Verification items for the finished model (mm, model axes). A direction names the side the tool comes from. Round coordinates to 2 decimals unless told otherwise and drop trailing zeros. Write each loop counter-clockwise with the first axis right and the second up, starting at its lowest first coordinate (ties: lowest second). Pieces come first, ordered by that corner, then holes. Notation, with made-up numbers: (45, -35.75) - (90, -35.75) arc R27 cw to (90, -3.75) - close; hole circle Ø9 at (26, 52.5). An arc over 180 degrees is marked (long way). Answer as a JSON object with one key per item and string values. Group by question number.
1) Set-up check for faces 4 (the flat face through (8.5, 10, 17)), 5 (the flat face through (2, 35, -11.5)): record each of +Z, -Z, +X, -X, +Y, -Y from which the full face is reachable in a straight line by a thin tool's end or side.
2) Section check C-C (x = 1.25). Enter the section's corners in (y, z).
3) Section check A-A (z = 18). Enter the section's corners in (x, y), then the cut area to 3 significant figures.
4) Thickness scan on line 1 (Y direction, x = 1.75, z = 0); line 2 (Y direction, x = -2.5, z = 0.5); line 3 (Z direction, x = -6.5, y = -2.5). Record the ranges inside material, lowest first.
5) Section check B-B (y = 42). Enter the section's corners in (x, z), then the cut area to 3 significant figures.
6) Mould release check, pull along Z, two halves, no side actions. Record for faces 1 (the cylindrical face through (0.119, -19.961, -10.382)), 2 (the flat face through (2, 35, 11.5)), 3 (the cylindrical face through (1.99, 34.11, -1.34)): +Z half, -Z half, draft (parallel to the pull), parting line (faces both ways), or undercut.
7) Section check D-D (z = 0). Enter the section's corners in (x, y), then the cut area to 3 significant figures.
8) Go/stop test with flat-tipped pins: pin 1 Ø2 at (x, z) = (5, 16) entering from +Y; pin 2 Ø3 at (x, z) = (-3.5, -6) entering from -Y; pin 3 Ø1.5 at (y, z) = (36.5, 5) entering from +X. Record where each tip stops, or that it passes through.
```python
from build123d import *

# Parameters (mm, degrees)
SKETCH2_R                = 22.5
BOSS_EXTRUDE1_DEPTH      = 8.5
BOSS_EXTRUDE2_REACH      = 78.386
BOSS_EXTRUDE2_END_RADIUS = 22.5
SKETCH3_W                = 10
SKETCH3_H                = 23
SKETCH8_R                = 2.5
CUT_EXTRUDE1_DEPTH       = 57.95722287
SKETCH11_R               = 19.5
CUT_EXTRUDE2_DEPTH       = 58.404268134


with BuildPart() as part:
    # Sketch2 → Boss-Extrude1 (new, symmetric)
    with BuildSketch(Plane(origin=(0, 0, 0), x_dir=(0, 0, -1), z_dir=(1, 0, 0))):
        Circle(SKETCH2_R)
    extrude(amount=BOSS_EXTRUDE1_DEPTH, both=True)

    # Boss-Extrude2: up to this cylinder (the profile starts outside it)
    boss_extrude2_end = Plane(origin=(1.923205, 0, 0), z_dir=(-1, 0, 0)) * Cylinder(BOSS_EXTRUDE2_END_RADIUS, 202.772, mode=Mode.PRIVATE)
    # Sketch3 → Boss-Extrude2 (add, up to the surface)
    with BuildSketch(Plane(origin=(0, 50, 0), x_dir=(1, 0, 0), z_dir=(0, 1, 0)), mode=Mode.PRIVATE) as boss_extrude2_sk1:
        with Locations((1.9232045, 0)):
            Rectangle(SKETCH3_W, SKETCH3_H)
    boss_extrude2_tool1 = extrude(boss_extrude2_sk1.sketch, amount=-BOSS_EXTRUDE2_REACH, mode=Mode.PRIVATE) - boss_extrude2_end
    add(boss_extrude2_tool1.solids().sort_by_distance((1.923205, 50, 0))[0])

    # Sketch8 → Cut-Extrude1 (cut, through all)
    with BuildSketch(Plane(origin=(6.9232045, 0, 0), x_dir=(0, 0, -1), z_dir=(1, 0, 0))):
        with Locations((0, 42)):
            Circle(SKETCH8_R)
        with Locations((0, 32)):
            Circle(SKETCH8_R)
    extrude(amount=-CUT_EXTRUDE1_DEPTH, mode=Mode.SUBTRACT)

    # Sketch11 → Cut-Extrude2 (cut, through all)
    with BuildSketch(Plane(origin=(8.5, 0, 0), x_dir=(0, 0, -1), z_dir=(1, 0, 0))):
        Circle(SKETCH11_R)
    extrude(amount=-CUT_EXTRUDE2_DEPTH, mode=Mode.SUBTRACT)


solid = part.part
```
Returned:
{
 "1": {"face 4": "+Z, -Z, +X, +Y, -Y", "face 5": "-Z, +X, -X, +Y"},
 "2": {"outline": "(19.34, -11.5) - (50, -11.5) - (50, 11.5) - (19.34, 11.5) arc R22.5 ccw (long way) to start; hole circle Ø39 at (0, 0); hole circle Ø5 at (32, 0); hole circle Ø5 at (42, 0)"},
 "3": {"outline": "(-8.5, -13.5) - (8.5, -13.5) - (8.5, -7.5) - (-8.5, -7.5) - close; (-8.5, 7.5) - (8.5, 7.5) - (8.5, 13.5) - (-8.5, 13.5) - close", "area": "204 mm2"},
 "4": {"line 1": "-22.5 to -19.5, 19.5 to 29.5, 34.5 to 39.5, 44.5 to 50", "line 2": "-22.49 to -19.49, 19.49 to 29.55, 34.45 to 39.55, 44.45 to 50", "line 3": "-22.36 to -19.34, 19.34 to 22.36"},
 "5": {"outline": "(-3.08, -11.5) - (6.92, -11.5) - (6.92, -2.5) - (-3.08, -2.5) - close; (-3.08, 2.5) - (6.92, 2.5) - (6.92, 11.5) - (-3.08, 11.5) - close", "area": "180 mm2"},
 "6": {"face 1": "parting line", "face 2": "+Z half", "face 3": "undercut"},
 "7": {"outline": "(-8.5, -22.5) - (8.5, -22.5) - (8.5, -19.5) - (-8.5, -19.5) - close; (-8.5, 19.5) - (8.5, 19.5) - (8.5, 22.5) - (6.92, 22.5) - (6.92, 29.5) - (-3.08, 29.5) - (-3.08, 22.5) - (-8.5, 22.5) - close; (-3.08, 34.5) - (6.92, 34.5) - (6.92, 39.5) - (-3.08, 39.5) - close; (-3.08, 44.5) - (6.92, 44.5) - (6.92, 50) - (-3.08, 50) - close", "area": "277 mm2"},
 "8": {"pin 1": "y = 16.77", "pin 2": "y = -22.05", "pin 3": "x = 6.92"}
}
